```python
from build123d import *

# Parameters (mm, degrees)
SKETCH1_R              = 4.5
SKETCH1_R_2            = 2.85
MAIN_AXIS_DEPTH        = 3
SKETCH2_W              = 10
SKETCH2_H              = 10
SKETCH2_R              = 1.5
BASE_OF_RECTAGLE_DEPTH = 1.3
SKETCH3_W              = 1.3
SKETCH3_H              = 10
PULLEY_SUPPORT_DEPTH   = 2


with BuildPart() as part:
    # Sketch1 → Main Axis (new body)
    with BuildSketch(Plane.XY):
        Circle(SKETCH1_R)
        Circle(SKETCH1_R_2, mode=Mode.SUBTRACT)
    extrude(amount=MAIN_AXIS_DEPTH)

    # Sketch2 → Base of Rectagle (add)
    with BuildSketch(Plane.XY.offset(3)):
        Rectangle(SKETCH2_W, SKETCH2_H)
        Circle(SKETCH2_R, mode=Mode.SUBTRACT)
    extrude(amount=BASE_OF_RECTAGLE_DEPTH)

    # Sketch3 → Pulley Support (add)
    with BuildSketch(Plane.XY.offset(4.3)):
        with Locations((-4.35, 0)):
            Rectangle(SKETCH3_W, SKETCH3_H)
        with Locations((4.35, 0)):
            Rectangle(SKETCH3_W, SKETCH3_H)
    extrude(amount=PULLEY_SUPPORT_DEPTH)


solid = part.part
```
Read the model definition and answer for the solid it produces. Units are mm, in the model's axes. A direction names the side the tool comes from. Coordinates: 2 decimals unless noted, no trailing zeros. Write each loop counter-clockwise with the first axis right and the second up, starting at its lowest first coordinate (ties: lowest second). Pieces come first, ordered by that corner, then holes. Notation, with made-up numbers: (15, 71) - (49, 71) arc R27 cw to (49, 95) - close; hole circle Ø2 at (0.25, 60). An arc over 180 degrees is marked (long way). Answer as a JSON object with one key per item and string values. Group by question number.
1. The mould has two halves that part along Y. Classify faces 1 (the flat face through (1.2, -1.2, 3)), 2 (the cylindrical face through (-2.262, -1.734, 1.479)), 3 (the flat face through (0, 5, 4)), 4 (the flat face through (3.7, 0, 5)): +Y half, -Y half, draft (parallel to the pull), parting line (faces both ways), or undercut.
2. Which of the six approach directions +Z, -Z, +X, -X, +Y, -Y give full straight-line access (tool end or side, diameter ignored) to faces 5 (the cylindrical face through (-1.5, 0.07, 3.64)), 6 (the flat face through (-3.7, 0, 5)), 7 (the flat face through (-1.2, 4.5, 3))?
3. A cutting plane is placed at B-B (z = 5). Determine the outline of the cut face in (x, y).
4. Consider L1, parallel to X at y = 3, z = 4.5; L2, parallel to Y at x = 0, z = 0.9; L3, parallel to Y at x = 0, z = 3.75. Determine where each line is inside the solid, lowest interval first. Write a range as [from, to].
5. A cutting plane is placed at A-A (x = 0). Determine the outline of the cut face in (y, z).
6. A cutting plane is placed at C-C (y = 0). Determine the outline of the cut face in (x, z).
7. A cutting plane is placed at D-D (z = 3.5). Determine the outline of the cut face in (x, y), plus the area to 3 significant figures.
8. Each of these flat-tipped pins is pushed along its axis until it touches: P1, Ø4.5, axis at x = -0.5, y = 0, coming from the -Z side; P2, Ø4, axis at x = 0, y = 0, coming from the +Z side. Where does it stop, or does it pass through?
Worked out:
{
 "1": {"face 1": "undercut", "face 2": "undercut", "face 3": "+Y half", "face 4": "draft"},
 "2": {"face 5": "+Z, -Z", "face 6": "+Z, +Y, -Y", "face 7": "-Z"},
 "3": {"outline": "(-5, -5) - (-3.7, -5) - (-3.7, 5) - (-5, 5) - close; (3.7, -5) - (5, -5) - (5, 5) - (3.7, 5) - close"},
 "4": {"L1": "x = [-5, -3.7], [3.7, 5]", "L2": "y = [-4.5, -2.85], [2.85, 4.5]", "L3": "y = [-5, -1.5], [1.5, 5]"},
 "5": {"outline": "(-5, 3) - (-4.5, 3) - (-4.5, 0) - (-2.85, 0) - (-2.85, 3) - (-1.5, 3) - (-1.5, 4.3) - (-5, 4.3) - close; (1.5, 3) - (2.85, 3) - (2.85, 0) - (4.5, 0) - (4.5, 3) - (5, 3) - (5, 4.3) - (1.5, 4.3) - close"},
 "6": {"outline": "(-5, 3) - (-4.5, 3) - (-4.5, 0) - (-2.85, 0) - (-2.85, 3) - (-1.5, 3) - (-1.5, 4.3) - (-3.7, 4.3) - (-3.7, 6.3) - (-5, 6.3) - close; (1.5, 3) - (2.85, 3) - (2.85, 0) - (4.5, 0) - (4.5, 3) - (5, 3) - (5, 6.3) - (3.7, 6.3) - (3.7, 4.3) - (1.5, 4.3) - close"},
 "7": {"outline": "(-5, -5) - (5, -5) - (5, 5) - (-5, 5) - close; hole circle Ø3 at (0, 0)", "area": "92.9 mm²"},
 "8": {"P1": "stops at z = 3", "P2": "stops at z = 4.3"}
}
